Check sheet for the modelled part. Datum: model origin and axes. Units: mm. A direction names the side the tool comes from. Coordinates: 2 decimals unless noted, no trailing zeros. Loops run counter-clockwise (first coordinate to the right, second up) from the corner with the lowest first, then second, coordinate; pieces in that order, holes last. Notation, with made-up numbers: M 22,-27 L 48,-27 A20 cw 48,-7 Z; hole C 54,-0.5 d8. An arc over 180 degrees is marked long. Return JSON: item names as keys, results as strings.
from build123d import *

# Parameters (mm, degrees)
SKETCH2_R   = 2.9499941
BASE_DEPTH  = 1.00000054
SKETCH4_R   = 1.27
DIODE_DEPTH = 5.08


with BuildPart() as part:
    # Sketch1 → Shell (revolve)
    with BuildSketch(Plane.XY, mode=Mode.PRIVATE) as shell_sk:
        with BuildLine():
            Line((-2.499995, 0), (-2.499995, 6.1900054))
            ThreePointArc((-2.499995, 6.1900054), (-1.767763417, 7.957768817), (0, 8.6900004))
            Line((0, 8.6900004), (0, 8.4360004))
            ThreePointArc((0, 8.4360004), (-1.588158295, 7.778163695), (-2.245995, 6.1900054))
            Line((-2.245995, 6.1900054), (-2.245995, 0))
            Line((-2.245995, 0), (-2.499995, 0))
        make_face()
    revolve(shell_sk.sketch.rotate(Axis((0, 9.12450042, 0), (0, -1, 0)), 270), axis=Axis((0, 9.12450042, 0), (0, -1, 0)))

    # Sketch2 → Base (add)
    with BuildSketch(Plane(origin=(0, 0, 0), x_dir=(1, 0, 0), z_dir=(0, 1, 0))):
        with Locations(Location((0, 0, 0), (0, 0, 270))):
            Circle(SKETCH2_R)
    extrude(amount=-BASE_DEPTH)

    # Sketch4 → Diode (add)
    with BuildSketch(Plane(origin=(0, 0, 0), x_dir=(1, 0, 0), z_dir=(0, 1, 0))):
        with Locations(Location((0, 0, 0), (0, 0, 270))):
            Circle(SKETCH4_R)
    extrude(amount=DIODE_DEPTH)


solid = part.part
1) Section check D-D on x = 2. Record the cut outline in (y, z).
Answers:
{"outline": "M -1,-2.17 L 0,-2.17 L 0,-1.5 L 6.19,-1.5 A1.5 ccw 6.19,1.5 L 0,1.5 L 0,2.17 L -1,2.17 Z; hole M 0,-1.02 L 6.19,-1.02 A1.02 ccw 6.19,1.02 L 0,1.02 Z"}
2) Section check A-A on z = 0. Record the cut outline in (x, y), then the cut area to 3 significant figures.
Answers:
{"outline": "M -2.95,-1 L 2.95,-1 L 2.95,0 L 2.5,0 L 2.5,6.19 A2.5 ccw -2.5,6.19 L -2.5,0 L -2.95,0 Z; hole M -2.25,0 L -1.27,0 L -1.27,5.08 L 1.27,5.08 L 1.27,0 L 2.25,0 L 2.25,6.19 A2.25 ccw -2.25,6.19 Z", "area": "23.8 mm²"}
3) Draft check along Y on faces 1 (the face through (1.26, 2.5, -0.17)), 2 (the face through (0, -1, 0)), 3 (the face through (-1.795, -0.493, -2.341)). Enter one of: +Y half, -Y half, draft (parallel to the pull), parting line (faces both ways), or undercut.
Answers:
{"face 1": "undercut", "face 2": "-Y half", "face 3": "draft"}
4) Section check B-B on x = 0. Record the cut outline in (y, z).
Answers:
{"outline": "M -1,-2.95 L 0,-2.95 L 0,-2.5 L 6.19,-2.5 A2.5 ccw 6.19,2.5 L 0,2.5 L 0,2.95 L -1,2.95 Z; hole M 0,-2.25 L 6.19,-2.25 A2.25 ccw 6.19,2.25 L 0,2.25 L 0,1.27 L 5.08,1.27 L 5.08,-1.27 L 0,-1.27 Z"}
5) Scan lines: line 1 along X through (y, z) = (2.25, 0); line 2 along Z through (x, y) = (0.1, 6); line 3 along Z through (x, y) = (0.85, 0.75). Record each from-to range of solid material in increasing order. Write a range as [from, to].
Answers:
{"line 1": "[-2.5, -2.25], [-1.27, 1.27], [2.25, 2.5]", "line 2": "[-2.5, -2.24], [2.24, 2.5]", "line 3": "[-2.35, -2.08], [-0.94, 0.94], [2.08, 2.35]"}
6) Go/stop test with flat-tipped pins: pin 1 Ø2 at (x, z) = (-1.5, -1) entering from +Y; pin 2 Ø2 at (x, y) = (-2, 0) entering from -Z; pin 3 Ø0.8 at (x, z) = (0, -0.5) entering from +Y. Record where each tip stops, or that it passes through.
Answers:
{"pin 1": "y = 8.56", "pin 2": "z = -2.78", "pin 3": "y = 8.69"}
7) Section check C-C on y = 1. Record the cut outline in (x, z), then the cut area to 3 significant figures.
Answers:
{"outline": "C 0,0 d5; C 0,0 d2.54; hole C 0,0 d4.49", "area": "8.85 mm²"}
8) Set-up check for faces 4 (the face through (-0.751, 3.138, 2.385)), 5 (the face through (0, 5.08, 0)): record each of +Z, -Z, +X, -X, +Y, -Y from which the full face is reachable in a straight line by a thin tool's end or side.
Answers:
{"face 4": "+Y", "face 5": "none"}
